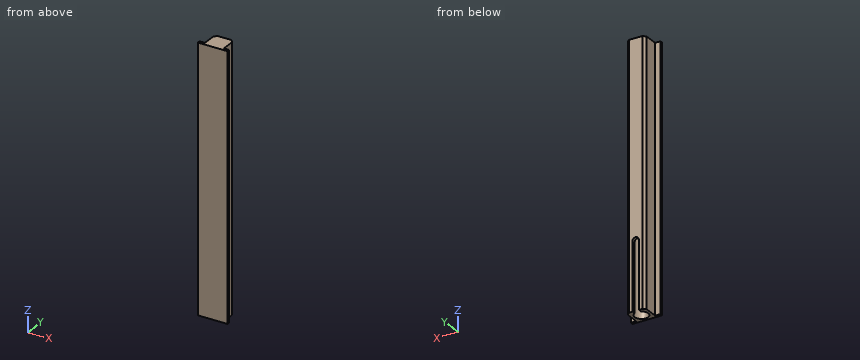
from build123d import *

# Parameters (mm, degrees)
F0_W     = 2
F0_H     = 1
F0_R     = 2.5
F1_DEPTH = 95
F3_DEPTH = 2
F5_SIZE  = 1
F6_SIZE  = 1
F7_W     = 2.4
F7_H     = 25
F8_DEPTH = 1.3078288801


with BuildPart() as f1:
    # F0 (on Top) → F1 (new body)
    with BuildSketch(Plane.XY):
        with Locations((-18.385866493, -45.4366366267)):
            Rectangle(F0_W, F0_H)
        Polygon((-10.385866493, -38.9366366267), (-17.385866493, -38.9366366267), (-17.385866493, -44.9366366267), (-17.385866493, -45.9366366267), (-10.385866493, -45.9366366267), (-10.385866493, -44.9366366267), align=None)
        with Locations((-13.885866493, -42.4366366267)):
            Circle(F0_R, mode=Mode.SUBTRACT)
        with Locations((-9.385866493, -45.4366366267)):
            Rectangle(F0_W, F0_H)
    extrude(amount=F1_DEPTH)


with BuildPart() as f3:
    # F2 (on face) → F3 (new body)
    with BuildSketch(Plane.XY.offset(95)):
        Polygon((-19.385866493, -44.9366366267), (-19.385866493, -45.9366366267), (-8.385866493, -45.9366366267), (-8.385866493, -44.9366366267), (-10.385866493, -44.9366366267), (-10.385866493, -38.9366366267), (-17.385866493, -38.9366366267), (-17.385866493, -44.9366366267), align=None)
    extrude(amount=F3_DEPTH)


with BuildPart() as f1_1:
    add(f1.part)

    # F4: union F3
    add(f3.part)

    # F5
    f5_edges = [f1_1.edges().sort_by_distance(p)[0] for p in [
        (-10.385866, -38.936637, 48.5),
    ]]
    chamfer(f5_edges, length=F5_SIZE)

    # F6
    f6_edges = [f1_1.edges().sort_by_distance(p)[0] for p in [
        (-17.385866, -38.936637, 48.5),
    ]]
    chamfer(f6_edges, length=F6_SIZE)

    # F7 (on face) → F8 (cut, through all)
    with BuildSketch(Plane(origin=(0, -38.9366366267, 0), x_dir=(-1, 0, 0), z_dir=(0, 1, 0))):
        with Locations((13.885866493, 12.5)):
            Rectangle(F7_W, F7_H)
        with BuildLine():
            ThreePointArc((15.085866493, 25), (13.885866493, 26.2), (12.685866493, 25))
            Line((12.685866493, 25), (15.085866493, 25))
        make_face()
    extrude(amount=-F8_DEPTH, mode=Mode.SUBTRACT)


solid = f1_1.part
Could you check a few things on this model? Use its own coordinates, in mm. Coordinates: 2 decimals unless noted, no trailing zeros. Order: outer loops, then holes, each group sorted by start corner. A loop starts at its lowest first (then second) coordinate and runs counter-clockwise, first axis right, second up.
Q1. Will these pins go through, and if not, where does the flat tip stop? pin 1 (1.5 mm diameter, centred on y = -43, z = 67.5, fed in from -X); pin 2 (0.6 mm diameter, centred on x = -18, z = 70, fed in from +Y); pin 3 (1.5 mm diameter, centred on y = -42, z = 48, fed in from +X); pin 4 (4 mm diameter, centred on x = -13.5, y = -43, fed in from -Z).
Q2. Suppose I cut it at A-A on z = 21. Please give me the cut outline in (x, y), and give its area (3 significant figures).
Q3. Please list where these lines run through material, in increasing order: L1, parallel to X at y = -42.75, z = 79; L2, parallel to Z at x = -14, y = -40.75; L3, parallel to Y at x = -16, z = 23.5.
Q4. Suppose I cut it at B-B on z = 72.5. Please give me the cut outline in (x, y).
Answer:
1. pin 1: stops at x = -17.39
1. pin 2: stops at y = -44.94
1. pin 3: stops at x = -10.39
1. pin 4: stops at z = 0
2. outline: (-19.39, -45.94) - (-8.39, -45.94) - (-8.39, -44.94) - (-10.39, -44.94) - (-10.39, -39.94) - (-11.39, -38.94) - (-12.69, -38.94) - (-12.69, -40.24) arc R2.5 cw (long way) to (-15.09, -40.24) - (-15.09, -38.94) - (-16.39, -38.94) - (-17.39, -39.94) - (-17.39, -44.94) - (-19.39, -44.94) - close
2. area: 29.7 mm2
3. L1: x = -17.39 to -16.37, -11.41 to -10.39
3. L2: z = 95 to 97
3. L3: y = -45.94 to -43.77, -41.1 to -38.94
4. outline: (-19.39, -45.94) - (-8.39, -45.94) - (-8.39, -44.94) - (-10.39, -44.94) - (-10.39, -39.94) - (-11.39, -38.94) - (-16.39, -38.94) - (-17.39, -39.94) - (-17.39, -44.94) - (-19.39, -44.94) - close; hole circle Ø5 at (-13.89, -42.44)
